Verification items for this drawing (mm, ordinates from the low corner). Coordinates: 2 decimals unless noted, no trailing zeros. Write each loop counter-clockwise with the first axis right and the second up, starting at its lowest first coordinate (ties: lowest second). Pieces come first, ordered by that corner, then holes. Notation, with made-up numbers: M 55,8.25 L 78,8.25 A20 ccw 78,41.25 Z; hole C 51,-25 d8. An arc over 180 degrees is marked long. Put each result on its own line as item: value. Start each with the question number.
1) Mould release check, pull along Z, two halves, no side actions. Record for the marked faces 1, 2 and 3: released by +Z, released by -Z, zero draft, split by the parting line, or undercut.
2) Cross-section at D-D on z = 16. Record the cut outline in (x, y), plus the area to 3 significant figures.
3) Gauge pin test, flat end, axial feed: pin 1 (1 mm diameter, centred on x = 59, z = 50, fed in from -Y). Record the tip position at first contact, or that the pin passes through.
4) Cross-section at A-A on x = 37. Record the cut outline in (y, z), plus the area to 3 significant figures.
5) Scan lines: line 1 along Z through (x, y) = (53, 13.5) (1 decimal); line 2 along Z through (x, y) = (40.5, 18.5) (1 decimal); line 3 along X through (y, z) = (33, 48). Record each from-to range of solid material in increasing order.
6) Cross-section at B-B on z = 33. Record the cut outline in (x, y) (1 decimal).
7) Cross-section at C-C on y = 4.5. Record the cut outline in (x, z), plus the area to 3 significant figures.
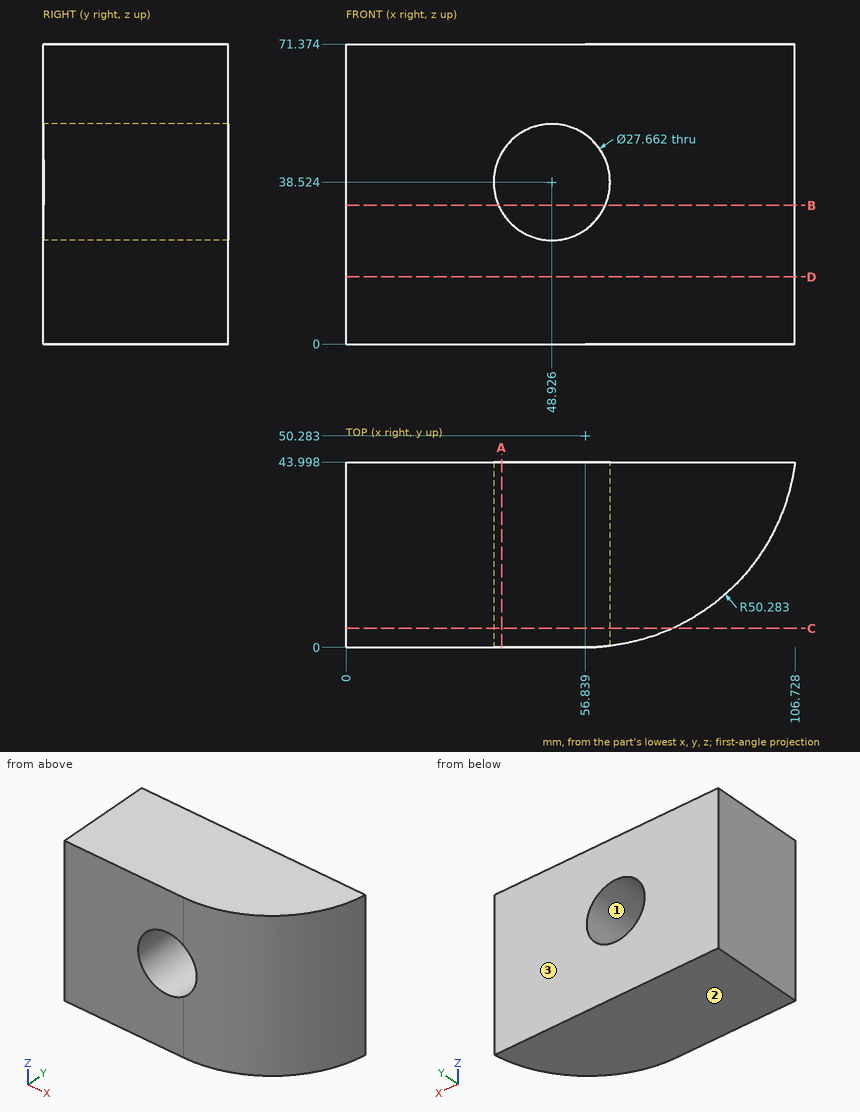
Answer key:
1. face 1: undercut
1. face 2: released by -Z
1. face 3: zero draft
2. outline: M 0,0 L 56.84,0 A50.28 ccw 106.73,44 L 0,44 Z
2. area: 4,170 mm²
3. pin 1: stops at y = 0.03
4. outline: M 0,0 L 44,0 L 44,31.52 L 0,31.52 Z; M 0,45.53 L 44,45.53 L 44,71.37 L 0,71.37 Z
4. area: 2,520 mm²
5. line 1: z = 0 to 25.3, 51.7 to 71.4
5. line 2: z = 0 to 27.6, 49.5 to 71.4
5. line 3: x = 0 to 38.85, 59 to 104.06
6. outline: M 0,0 L 36.2,0 L 36.2,44 L 0,44 Z; M 61.6,0.2 A50.3 ccw 106.7,44 L 61.6,44 Z
7. outline: M 0,0 L 77.63,0 L 77.63,71.37 L 0,71.37 Z; hole C 48.93,38.52 d27.66
7. area: 4,940 mm²
